Read the model definition and answer for the solid it produces. Units are mm, in the model's axes. Face numbers are marked on the shaded views. Give positions to 0.01 mm unless a question says otherwise; leave off trailing zeros. Write each loop counter-clockwise with the first axis right and the second up, starting at its lowest first coordinate (ties: lowest second). Pieces come first, ordered by that corner, then holes. Notation, with made-up numbers: (29.5, -1.75) -> (55.5, -1.75) arc R27 cw to (55.5, 26.25) -> close; hole circle Ø5 at (29, 81). An arc over 180 degrees is marked (long way). Use a Markdown table: item, result.
from build123d import *

# Parameters (mm, degrees)
SKETCH1_R          = 171.45
EXTRUDE1_DEPTH     = 36.5125
SKETCH2_R          = 11.1125
EXTRUDE2_DEPTH     = 246.20066814
CIRPATTERN1_COUNT  = 8
FILLET1_R          = 1.154545455
SKETCH5_R          = 72
CUT_EXTRUDE1_DEPTH = 237.236


with BuildPart() as part:
    # Sketch1 → Extrude1 (new body)
    with BuildSketch(Plane.XY):
        Circle(SKETCH1_R)
    extrude(amount=EXTRUDE1_DEPTH)

    # Sketch2 → Extrude2 (cut, through all)
    with BuildSketch(Plane.XY.offset(36.5125)):
        with Locations((0, 149.225)):
            Circle(SKETCH2_R)
    extrude2 = extrude(amount=-EXTRUDE2_DEPTH, mode=Mode.SUBTRACT)

    # CirPattern1: Extrude2 ×8 about axis
    cirpattern1_axis = Axis((0, 0, 0), (0, 0, 1))
    for i in range(1, CIRPATTERN1_COUNT):
        add(extrude2.rotate(cirpattern1_axis, i * 360 / CIRPATTERN1_COUNT), mode=Mode.SUBTRACT)

    # Sketch3 → Cut-Revolve1 (revolve, cut)
    with BuildSketch(Plane(origin=(0, 0, 0), x_dir=(0, 0, -1), z_dir=(1, 0, 0))):
        Polygon((-36.5125, 109.9185), (-18.25625, 109.347), (-18.25625, 0), (-36.5125, 0), align=None)
    revolve(axis=Axis((0, 0, 18.25625), (0, 0, 1)), mode=Mode.SUBTRACT)

    # Fillet1
    fillet1_edges = [part.edges().sort_by_distance(p)[0] for p in [
        (0, -109.347, 18.25625),
        (0, -109.9185, 36.5125),
        (-171.45, 0, 36.5125),
    ]]
    fillet(fillet1_edges, radius=FILLET1_R)

    # Sketch5 → Cut-Extrude1 (cut)
    with BuildSketch(Plane(origin=(0, 0, 0), x_dir=(-1, 0, 0), z_dir=(0, 0, -1))):
        Circle(SKETCH5_R)
    extrude(amount=-CUT_EXTRUDE1_DEPTH, mode=Mode.SUBTRACT)


solid = part.part
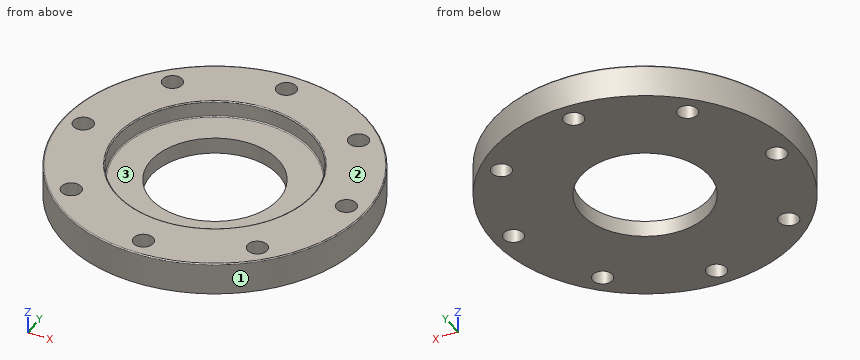
Item 1: Each of these flat-tipped pins is pushed along its axis until it touches: P1, Ø3, axis at y = 63.5, z = 12.5, coming from the +X side; P2, Ø3, axis at x = -66, z = 12, coming from the -Y side; P3, Ø2, axis at y = 17, z = 17, coming from the +X side. Where does it stop, or does it pass through?
Return value:
| item | result |
|---|---|
| P1 | x = 159.85 |
| P2 | y = -158.85 |
| P3 | x = 170.7 |
Item 2: A cutting plane is placed at C-C (z = 9.5). Count the separate pieces of the cut face and the enclosed holes in it, then the cut area to 3 significant figures.
Return value:
| item | result |
|---|---|
| separate pieces | 1 |
| enclosed holes | 9 |
| area | 73,000 mm^2 |
Item 3: Straight lines are drawn through the part: line 1 along Y through (x, z) = (0, 18); line 2 along Y through (x, z) = (0, 27); line 3 along X through (y, z) = (106, 5). For each, find the intervals that lie inside material, in ascending order. Write a range as [from, to].
Return value:
| item | result |
|---|---|
| line 1 | [-171.45, -160.34], [-138.11, -72], [72, 138.11], [160.34, 171.45] |
| line 2 | [-171.45, -160.34], [-138.11, -109.62], [109.62, 138.11], [160.34, 171.45] |
| line 3 | [-134.76, -116.62], [-94.42, 94.42], [116.62, 134.76] |
Item 4: For a pull along X with two mould halves and no side action, classify the marked faces 1, 2 and 3 as +X half, -X half, draft (parallel to the pull), parting line (faces both ways), or undercut.
Return value:
| item | result |
|---|---|
| face 1 | parting line |
| face 2 | draft |
| face 3 | undercut |
Item 5: A cutting plane is placed at A-A (x = 0). Give the vertices of the cut face in (y, z).
Return value:
| item | result |
|---|---|
| outline | (-171.45, 0) -> (-160.34, 0) -> (-160.34, 36.51) -> (-170.3, 36.51) arc R1.15 ccw to (-171.45, 35.36) -> close; (-138.11, 0) -> (-72, 0) -> (-72, 18.26) -> (-108.23, 18.26) arc R1.15 cw to (-109.38, 19.37) -> (-109.88, 35.39) arc R1.15 ccw to (-111.04, 36.51) -> (-138.11, 36.51) -> close; (72, 0) -> (138.11, 0) -> (138.11, 36.51) -> (111.04, 36.51) arc R1.15 ccw to (109.88, 35.39) -> (109.38, 19.37) arc R1.15 cw to (108.23, 18.26) -> (72, 18.26) -> close; (160.34, 0) -> (171.45, 0) -> (171.45, 35.36) arc R1.15 ccw to (170.3, 36.51) -> (160.34, 36.51) -> close |
